from build123d import *

# Parameters (mm, degrees)
SKETCH1_R              = 50
BOSS_EXTRUDE1_DEPTH    = 3
SPLIT1_SURFACE_1_BACK  = 170.732
SPLIT1_SURFACE_1_DEPTH = 341.464
SPLIT1_SURFACE_2_BACK  = 170.732
SPLIT1_SURFACE_2_DEPTH = 341.464
BODY_DELETE1_DEPTH     = 3
FILLET1_R              = 3
BOSS_EXTRUDE4_DEPTH    = 3
SPLIT2_SURFACE_3_BACK  = 109.724
SPLIT2_SURFACE_3_DEPTH = 219.448
SPLIT2_SURFACE_4_BACK  = 109.724
SPLIT2_SURFACE_4_DEPTH = 219.448
FILLET2_R              = 3
SKETCH5_R              = 1
CUT_EXTRUDE1_DEPTH     = 3
SKETCH6_W              = 8
SKETCH6_H              = 5
BOSS_EXTRUDE5_DEPTH    = 3
SKETCH7_W              = 5
SKETCH7_H              = 4
CUT_EXTRUDE2_DEPTH     = 3


# Read off the part's stored shape, not the designer's step: Body-Delete1
with BuildPart() as part:
    # Sketch1 → Boss-Extrude1 (new body)
    with BuildSketch(Plane(origin=(0, 0, 0), x_dir=(1, 0, 0), z_dir=(0, 1, 0))):
        with BuildLine():
            ThreePointArc((10, 0), (-107.445626465, 17.320508076), (0, -33.166247904))
            Line((0, -33.166247904), (0, -60))
            Line((0, -60), (10, -60))
            Line((10, -60), (10, 0))
        make_face()
        with Locations(Location((-50, 0, 0), (0, 0, 270))):
            Circle(SKETCH1_R, mode=Mode.SUBTRACT)
    extrude(amount=BOSS_EXTRUDE1_DEPTH)


with BuildPart() as body_2:
    # Split1: the piece behind the surface
    add(part.part)
    # Split1 surface: a surface, the sketch's curves swept straight by 341.464 mm
    with BuildLine(Plane(origin=(0, 3, 0), x_dir=(1, 0, 0), z_dir=(0, 1, 0)).offset(-SPLIT1_SURFACE_1_BACK), mode=Mode.PRIVATE) as split1_surface_1_path:
        Line((0, -33.166247904), (0, 0))
        Line((0, 0), (-12, 0))
        Line((-12, 0), (-12, 32.496153619))
        Line((-12, 32.496153619), (-12, 67.159700612))
        Line((-12, 67.159700612), (-127.638562935, 67.159700612))
        Line((-127.638562935, 67.159700612), (-127.638562935, -72.196904976))
        Line((-127.638562935, -72.196904976), (0, -72.196904976))
        Line((0, -72.196904976), (0, -33.166247904))
    split1_surface_1 = Shell.extrude(split1_surface_1_path.wire(), (0 * SPLIT1_SURFACE_1_DEPTH, 1 * SPLIT1_SURFACE_1_DEPTH, 0 * SPLIT1_SURFACE_1_DEPTH))
    split(bisect_by=split1_surface_1, keep=Keep.BOTTOM)

    # Fillet1
    fillet1_edges = [body_2.edges().sort_by_distance(p)[0] for p in [
        (10, 1.5, 60),
    ]]
    fillet(fillet1_edges, radius=FILLET1_R)

    # Sketch3 → Boss-Extrude4 (add)
    with BuildSketch(Plane(origin=(0, 3, 0), x_dir=(1, 0, 0), z_dir=(0, 1, 0))):
        Polygon((0, -50), (-8, -50), (-8, -40), (0, -40), (3, -40), (3, -50), align=None)
        Polygon((-8, -20), (-8, -30), (0, -30), (3, -30), (3, -20), (0, -20), align=None)
    extrude(amount=-BOSS_EXTRUDE4_DEPTH)


with BuildPart() as part_1:
    add(part.part)

    # Split1: split by a surface, the side it looks to stays
    # Split1 surface: a surface, the sketch's curves swept straight by 341.464 mm
    with BuildLine(Plane(origin=(0, 3, 0), x_dir=(1, 0, 0), z_dir=(0, 1, 0)).offset(-SPLIT1_SURFACE_2_BACK), mode=Mode.PRIVATE) as split1_surface_2_path:
        Line((0, -33.166247904), (0, 0))
        Line((0, 0), (-12, 0))
        Line((-12, 0), (-12, 32.496153619))
        Line((-12, 32.496153619), (-12, 67.159700612))
        Line((-12, 67.159700612), (-127.638562935, 67.159700612))
        Line((-127.638562935, 67.159700612), (-127.638562935, -72.196904976))
        Line((-127.638562935, -72.196904976), (0, -72.196904976))
        Line((0, -72.196904976), (0, -33.166247904))
    split1_surface_2 = Shell.extrude(split1_surface_2_path.wire(), (0 * SPLIT1_SURFACE_2_DEPTH, 1 * SPLIT1_SURFACE_2_DEPTH, 0 * SPLIT1_SURFACE_2_DEPTH))
    split(bisect_by=split1_surface_2, keep=Keep.TOP)

    # Body-Delete1 outline → Body-Delete1 (cut)
    with BuildSketch(Plane(origin=(0, 0, 0), x_dir=(1, 0, 0), z_dir=(0, 1, 0))):
        with BuildLine():
            ThreePointArc((-12, 46.432747065), (-109.329587897, -8.94427191), (0, -33.166247904))
            Line((0, -33.166247904), (0, 0))
            ThreePointArc((0, 0), (-96.904157598, -17.320508075), (-12, 32.496153619))
            Line((-12, 32.496153619), (-12, 46.432747065))
        make_face()
    extrude(amount=BODY_DELETE1_DEPTH, mode=Mode.SUBTRACT)


with BuildPart() as body_2_2:
    # Split2: the piece behind the surface
    add(body_2.part)
    # Split2 surface: a surface, the sketch's curves swept straight by 219.448 mm
    with BuildLine(Plane(origin=(0, 3, 0), x_dir=(1, 0, 0), z_dir=(0, 1, 0)).offset(-SPLIT2_SURFACE_3_BACK), mode=Mode.PRIVATE) as split2_surface_3_path:
        Line((-12, 40.432747065), (-5.669502994, 40.432747065))
        Line((-5.669502994, 40.432747065), (-5.042290504, 40.432747065))
        Line((-5.042290504, 40.432747065), (-5.042290504, 47.453598883))
        Line((-5.042290504, 47.453598883), (-14.646815791, 47.453598883))
        Line((-14.646815791, 47.453598883), (-14.646815791, 40.432747065))
        Line((-14.646815791, 40.432747065), (-12, 40.432747065))
    split2_surface_3 = Shell.extrude(split2_surface_3_path.wire(), (0 * SPLIT2_SURFACE_3_DEPTH, 1 * SPLIT2_SURFACE_3_DEPTH, 0 * SPLIT2_SURFACE_3_DEPTH))
    split(bisect_by=split2_surface_3, keep=Keep.BOTTOM)

    # Fillet2
    fillet2_edges = [body_2_2.edges().sort_by_distance(p)[0] for p in [
        (-5.669502994, 1.5, -40.432747065),
    ]]
    fillet(fillet2_edges, radius=FILLET2_R)

    # Sketch5 → Cut-Extrude1 (cut)
    with BuildSketch(Plane(origin=(0, 3, 0), x_dir=(1, 0, 0), z_dir=(0, 1, 0))):
        with Locations(Location((-10, 38.432747065, 0), (0, 0, 270))):
            Circle(SKETCH5_R)
        with Locations(Location((-7, 35.432747065, 0), (0, 0, 270))):
            Circle(SKETCH5_R)
    extrude(amount=-CUT_EXTRUDE1_DEPTH, mode=Mode.SUBTRACT)

    # Sketch6 → Boss-Extrude5 (add)
    with BuildSketch(Plane(origin=(0, 3, 0), x_dir=(1, 0, 0), z_dir=(0, 1, 0))):
        with Locations((-1, -39.5)):
            Rectangle(SKETCH6_W, SKETCH6_H)
        with Locations((-1, -50.5)):
            Rectangle(SKETCH6_W, SKETCH6_H)
        with Locations((-1, -19.5)):
            Rectangle(SKETCH6_W, SKETCH6_H)
        with Locations((-1, -30.5)):
            Rectangle(SKETCH6_W, SKETCH6_H)
    extrude(amount=-BOSS_EXTRUDE5_DEPTH)

    # Sketch7 → Cut-Extrude2 (cut)
    with BuildSketch(Plane(origin=(0, 3, 0), x_dir=(1, 0, 0), z_dir=(0, 1, 0))):
        with Locations((-2.5, -25)):
            Rectangle(SKETCH7_W, SKETCH7_H)
        with Locations((-2.5, -45)):
            Rectangle(SKETCH7_W, SKETCH7_H)
    extrude(amount=-CUT_EXTRUDE2_DEPTH, mode=Mode.SUBTRACT)


with BuildPart() as body_2_1:
    add(body_2.part)

    # Split2: split by a surface, the side it looks to stays
    # Split2 surface: a surface, the sketch's curves swept straight by 219.448 mm
    with BuildLine(Plane(origin=(0, 3, 0), x_dir=(1, 0, 0), z_dir=(0, 1, 0)).offset(-SPLIT2_SURFACE_4_BACK), mode=Mode.PRIVATE) as split2_surface_4_path:
        Line((-12, 40.432747065), (-5.669502994, 40.432747065))
        Line((-5.669502994, 40.432747065), (-5.042290504, 40.432747065))
        Line((-5.042290504, 40.432747065), (-5.042290504, 47.453598883))
        Line((-5.042290504, 47.453598883), (-14.646815791, 47.453598883))
        Line((-14.646815791, 47.453598883), (-14.646815791, 40.432747065))
        Line((-14.646815791, 40.432747065), (-12, 40.432747065))
    split2_surface_4 = Shell.extrude(split2_surface_4_path.wire(), (0 * SPLIT2_SURFACE_4_DEPTH, 1 * SPLIT2_SURFACE_4_DEPTH, 0 * SPLIT2_SURFACE_4_DEPTH))
    split(bisect_by=split2_surface_4, keep=Keep.TOP)


solid = body_2_2.part
Verification items for the finished model (mm, model axes). A direction names the side the tool comes from. Coordinates: 2 decimals unless noted, no trailing zeros. Loops run counter-clockwise (first coordinate to the right, second up) from the corner with the lowest first, then second, coordinate; pieces in that order, holes last. Notation, with made-up numbers: (10.25, 61.5) -> (20.25, 61.5) arc R23 cw to (20.25, 95.5) -> close; hole circle Ø5 at (15.5, 84). An arc over 180 degrees is marked (long way). Answer as a JSON object with one key per item and string values. Group by question number.
Item 1: Scan lines: probe 1 along Z at (x, y) = (-4, 2.45); probe 2 along X at (y, z) = (0.5, 56.5); probe 3 along Z at (x, y) = (-7.5, 2.85). Record each from-to range of solid material in increasing order.
Item 2: Sectioned sample at D-D on z = 14.5. Record the boundary of the cut face in (x, y).
Item 3: Depth check by flat-ended pin: pin 1 (0.9 mm diameter, centred on y = 2, z = 31.5, fed in from -X); pin 2 (1.5 mm diameter, centred on x = -3, y = 2, fed in from -Z); pin 3 (1 mm diameter, centred on y = 1, z = 11, fed in from -X). Enter the tip coordinate at first touch or a pass-through.
Item 4: Sectioned sample at C-C on y = 1.1. State how many separate pieces and enclosed holes the cut face has, plus the area to 3 significant figures.
Item 5: Sectioned sample at B-B on z = 45.5. Record the boundary of the cut face in (x, y), plus the area to 3 significant figures.
Item 6: Tool access check on faces 1 (the flat face through (-6, 2, 40)), 2 (the flat face through (2, 0, 9)), 3 (the flat face through (-3, 2, 27)), 4 (the flat face through (-3, 2, 53)). Record the directions out of +Z, -Z, +X, -X, +Y, -Y that give a thin tool (end or side, any length) a straight path to the whole face; none if there is none.
Item 7: Sectioned sample at A-A on x = -10. Record the boundary of the cut face in (y, z).
Evaluation:
{
 "1": {"probe 1": "z = -38.52 to -19.6, 17 to 23, 27 to 33, 37 to 43, 47 to 53", "probe 2": "x = 0 to 10", "probe 3": "z = -40.43 to -36.3, -34.57 to -26.34, 20 to 30, 40 to 50"},
 "2": {"outline": "(0, 0) -> (10, 0) -> (10, 3) -> (0, 3) -> close"},
 "3": {"pin 1": "stops at x = -5", "pin 2": "stops at z = -38.22", "pin 3": "stops at x = 0"},
 "4": {"separate pieces": "1", "enclosed holes": "4", "area": "1,200 mm²"},
 "5": {"outline": "(-8, 0) -> (-5, 0) -> (-5, 3) -> (-8, 3) -> close; (0, 0) -> (10, 0) -> (10, 3) -> (0, 3) -> close", "area": "39.0 mm²"},
 "6": {"face 1": "-X, +Y, -Y", "face 2": "+Z, -Z, +X, -X, -Y", "face 3": "+Y, -Y", "face 4": "+Z, -X, +Y, -Y"},
 "7": {"outline": "(0, -40.43) -> (3, -40.43) -> (3, -39.43) -> (0, -39.43) -> close; (0, -37.43) -> (3, -37.43) -> (3, -30) -> (0, -30) -> close"}
}
